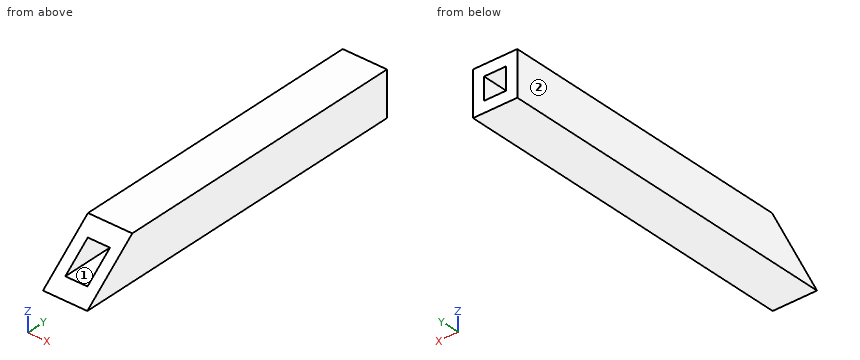
from build123d import *

# Parameters (mm, degrees)
SKETCH2_W           = 25.4
SKETCH2_H           = 203.2
BOSS_EXTRUDE2_DEPTH = 25.4
SKETCH3_W           = 12.7
SKETCH3_H           = 12.7
CUT_EXTRUDE1_DEPTH  = 207.350575478
CUT_EXTRUDE2_DEPTH  = 207.350575478


with BuildPart() as part:
    # Sketch2 → Boss-Extrude2 (new body)
    with BuildSketch(Plane.XY):
        with Locations((12.7, 101.6)):
            Rectangle(SKETCH2_W, SKETCH2_H)
    extrude(amount=BOSS_EXTRUDE2_DEPTH)

    # Sketch3 → Cut-Extrude1 (cut, through all)
    with BuildSketch(Plane.XZ):
        with Locations((12.7, 12.7)):
            Rectangle(SKETCH3_W, SKETCH3_H)
    extrude(amount=-CUT_EXTRUDE1_DEPTH, mode=Mode.SUBTRACT)

    # Sketch4 → Cut-Extrude2 (cut, through all)
    with BuildSketch(Plane(origin=(25.4, 0, 0), x_dir=(0, 0, -1), z_dir=(1, 0, 0))):
        Polygon((0, 0), (-25.4, 30.48), (-25.4, 0), align=None)
    extrude(amount=-CUT_EXTRUDE2_DEPTH, mode=Mode.SUBTRACT)


solid = part.part
Check sheet for the modelled part. Datum: model origin and axes. Units: mm. Face numbers are marked on the shaded views. A direction names the side the tool comes from. Give positions to 0.01 mm unless a question says otherwise; leave off trailing zeros. Order: outer loops, then holes, each group sorted by start corner. A loop starts at its lowest first (then second) coordinate and runs counter-clockwise, first axis right, second up. Notation, with made-up numbers: M 56.5,13 L 115.5,13 A25 ccw 115.5,25 Z; hole C -30,-39 d11. An arc over 180 degrees is marked long. Answer as CSV lines item,"result". Start each with the question number.
Item 1: Cross-section at C-C on y = 186. Enter the section's corners in (x, z).
Item 2: Tool access check on the marked faces 1 and 2. Record the directions out of +Z, -Z, +X, -X, +Y, -Y that give a thin tool (end or side, any length) a straight path to the whole face; none if there is none.
Item 3: Cross-section at B-B on z = 13.25. Enter the section's corners in (x, y), plus the area to 3 significant figures.
Item 4: Cross-section at A-A on x = 14. Enter the section's corners in (y, z), plus the area to 3 significant figures.
Item 5: Cross-section at D-D on z = 22.25. Enter the section's corners in (x, y).
Item 6: Gauge pin test, flat ends, axial feed: P1, Ø4, axis at x = 13, y = 71.5, coming from the -Z side; P2, Ø4, axis at x = 3, z = 6, coming from the -Y side. Record the tip position at first contact, or that the pin passes through.
Item 7: Thickness scan on line 1 (Z direction, x = 18.5, y = 68.5); line 2 (Y direction, x = 23, z = 18.5). Record the ranges inside material, lowest first. Write a range as [from, to].
Established:
1,outline,"M 0,0 L 25.4,0 L 25.4,25.4 L 0,25.4 Z; hole M 6.35,6.35 L 19.05,6.35 L 19.05,19.05 L 6.35,19.05 Z"
2,face 1,"+Y, -Y"
2,face 2,"+Z, -Z, -X, +Y, -Y"
3,outline,"M 0,15.9 L 6.35,15.9 L 6.35,203.2 L 0,203.2 Z; M 19.05,15.9 L 25.4,15.9 L 25.4,203.2 L 19.05,203.2 Z"
3,area,"2,380 mm^2"
4,outline,"M 0,0 L 203.2,0 L 203.2,6.35 L 7.62,6.35 Z; M 22.86,19.05 L 203.2,19.05 L 203.2,25.4 L 30.48,25.4 Z"
4,area,"2,390 mm^2"
5,outline,"M 0,26.7 L 25.4,26.7 L 25.4,203.2 L 0,203.2 Z"
6,P1,"stops at z = 0"
6,P2,"stops at y = 4.8"
7,line 1,"z = [0, 6.35], [19.05, 25.4]"
7,line 2,"y = [22.2, 203.2]"
